The listing builds one solid part. Answer for the finished solid, in the listing's coordinates (mm). A direction names the side the tool comes from. Round coordinates to 2 decimals unless told otherwise and drop trailing zeros. Write each loop counter-clockwise with the first axis right and the second up, starting at its lowest first coordinate (ties: lowest second). Pieces come first, ordered by that corner, then holes.
from build123d import *

# Parameters (mm, degrees)
SKETCH_1_R               = 1.75
SKETCH_1_R_2             = 2.5
EXTRUDE_1_DEPTH          = 4
SKETCH_2_R               = 1.75
CUT_EXTRUDE_1_DEPTH      = 4
PATTERN_CIRCULAR_1_COUNT = 4
SKETCH_4_R               = 10.25
CUT_EXTRUDE_2_DEPTH      = 2.5


with BuildPart() as part:
    # 草图1 → 凸台-拉伸1 (new body)
    with BuildSketch(Plane(origin=(0, 0, 0), x_dir=(0, 0, -1), z_dir=(1, 0, 0))):
        with BuildLine():
            Line((-4.841229183, 31.25), (-12.103072957, 3.125))
            ThreePointArc((-12.103072957, 3.125), (0, -12.5), (12.103072957, 3.125))
            Line((12.103072957, 3.125), (4.841229183, 31.25))
            ThreePointArc((4.841229183, 31.25), (0, 35), (-4.841229183, 31.25))
        make_face()
        with Locations((0, 30)):
            Circle(SKETCH_1_R, mode=Mode.SUBTRACT)
        Circle(SKETCH_1_R_2, mode=Mode.SUBTRACT)
    extrude(amount=EXTRUDE_1_DEPTH)

    # 草图2 → 切除-拉伸1 (cut)
    with BuildSketch(Plane(origin=(4, 0, 0), x_dir=(0, 0, -1), z_dir=(1, 0, 0))):
        with Locations((0, -7)):
            Circle(SKETCH_2_R)
    cut_extrude_1 = extrude(amount=-CUT_EXTRUDE_1_DEPTH, mode=Mode.SUBTRACT)

    # 阵列(圆周)1: 切除-拉伸1 ×4 about axis
    pattern_circular_1_axis = Axis((0, 0, 0), (1, 0, 0))
    for i in range(1, PATTERN_CIRCULAR_1_COUNT):
        add(cut_extrude_1.rotate(pattern_circular_1_axis, i * 360 / PATTERN_CIRCULAR_1_COUNT), mode=Mode.SUBTRACT)

    # 草图4 → 切除-拉伸2 (cut)
    with BuildSketch(Plane.ZY):
        Circle(SKETCH_4_R)
    extrude(amount=-CUT_EXTRUDE_2_DEPTH, mode=Mode.SUBTRACT)


solid = part.part
1. Straight lines are drawn through the part: line 1 along Z through (x, y) = (3.55, 0); line 2 along Y through (x, z) = (0.9, -1); line 3 along Z through (x, y) = (0.6, 6). For each, find the intervals that lie inside material, in ascending order.
Geometry says:
line 1: z = -12.5 to -8.75, -5.25 to -2.5, 2.5 to 5.25, 8.75 to 12.5
line 2: y = -12.46 to -10.2, 10.2 to 28.56, 31.44 to 34.9
line 3: z = -11.36 to -8.31, 8.31 to 11.36
2. Section A-A on z = 0 is taken. Determine the outline of the cut face in (x, y).
Geometry says:
outline: (0, -12.5) - (4, -12.5) - (4, -8.75) - (2.5, -8.75) - (2.5, -10.25) - (0, -10.25) - close; (0, 10.25) - (2.5, 10.25) - (2.5, 8.75) - (4, 8.75) - (4, 28.25) - (0, 28.25) - close; (0, 31.75) - (4, 31.75) - (4, 35) - (0, 35) - close; (2.5, -5.25) - (4, -5.25) - (4, -2.5) - (2.5, -2.5) - close; (2.5, 2.5) - (4, 2.5) - (4, 5.25) - (2.5, 5.25) - close
3. Section C-C on y = 6.5 is taken. Determine the outline of the cut face in (x, z).
Geometry says:
outline: (0, -11.23) - (4, -11.23) - (4, -1.68) - (2.5, -1.68) - (2.5, -7.93) - (0, -7.93) - close; (0, 7.93) - (2.5, 7.93) - (2.5, 1.68) - (4, 1.68) - (4, 11.23) - (0, 11.23) - close
4. Given pin 1 (12 mm diameter, centred on y = 28.5, z = 1.5, fed in from -X); pin 2 (1 mm diameter, centred on x = 2, y = 29.5, fed in from +Z); pin 3 (1 mm diameter, centred on x = 2, y = 21, fed in from -Z); pin 4 (4.5 mm diameter, centred on y = -7, z = 0, fed in from -X), each flat-ended and moving along its own axis, determine where each tip first touches the part or whether it passes through.
Geometry says:
pin 1: stops at x = 0
pin 2: stops at z = 5.42
pin 3: stops at z = -7.62
pin 4: stops at x = 2.5
5. Section D-D on x = 0.7 is taken. Determine the outline of the cut face in (y, z) (3 decimals).
Geometry says:
outline: (3.125, -12.103) - (31.25, -4.841) arc R5 ccw to (31.25, 4.841) - (3.125, 12.103) arc R12.5 ccw (long way) to start; hole circle Ø20.5 at (0, 0); hole circle Ø3.5 at (30, 0)
6. Section B-B on x = 3.1 is taken. Determine the outline of the cut face in (y, z) (3 decimals), plus the area to 3 significant figures.
Geometry says:
outline: (3.125, -12.103) - (31.25, -4.841) arc R5 ccw to (31.25, 4.841) - (3.125, 12.103) arc R12.5 ccw (long way) to start; hole circle Ø3.5 at (-7, 0); hole circle Ø5 at (0, 0); hole circle Ø3.5 at (0, -7); hole circle Ø3.5 at (0, 7); hole circle Ø3.5 at (7, 0); hole circle Ø3.5 at (30, 0)
area: 758 mm2
7. A tool of negligible diameter and unlimited length cuts with its end or side. For faces 4 (the face through (3.26, 8.71, -0.38)), 5 (the face through (1.232, -10.006, -2.222)), from which of +Z, -Z, +X, -X, +Y, -Y can it reach the whole face along a straight path? Write none if from no direction.
Geometry says:
face 4: +X, -X
face 5: -X
8. For a pull along Z with two mould halves and no side action, classify faces 1 (the face through (2, 35, 0)), 2 (the face through (2.5, -2, 2)), 3 (the face through (1.972, 16.991, -8.523)) as released by +Z, released by -Z, zero draft, split by the parting line, or undercut.
Geometry says:
face 1: split by the parting line
face 2: undercut
face 3: released by -Z
